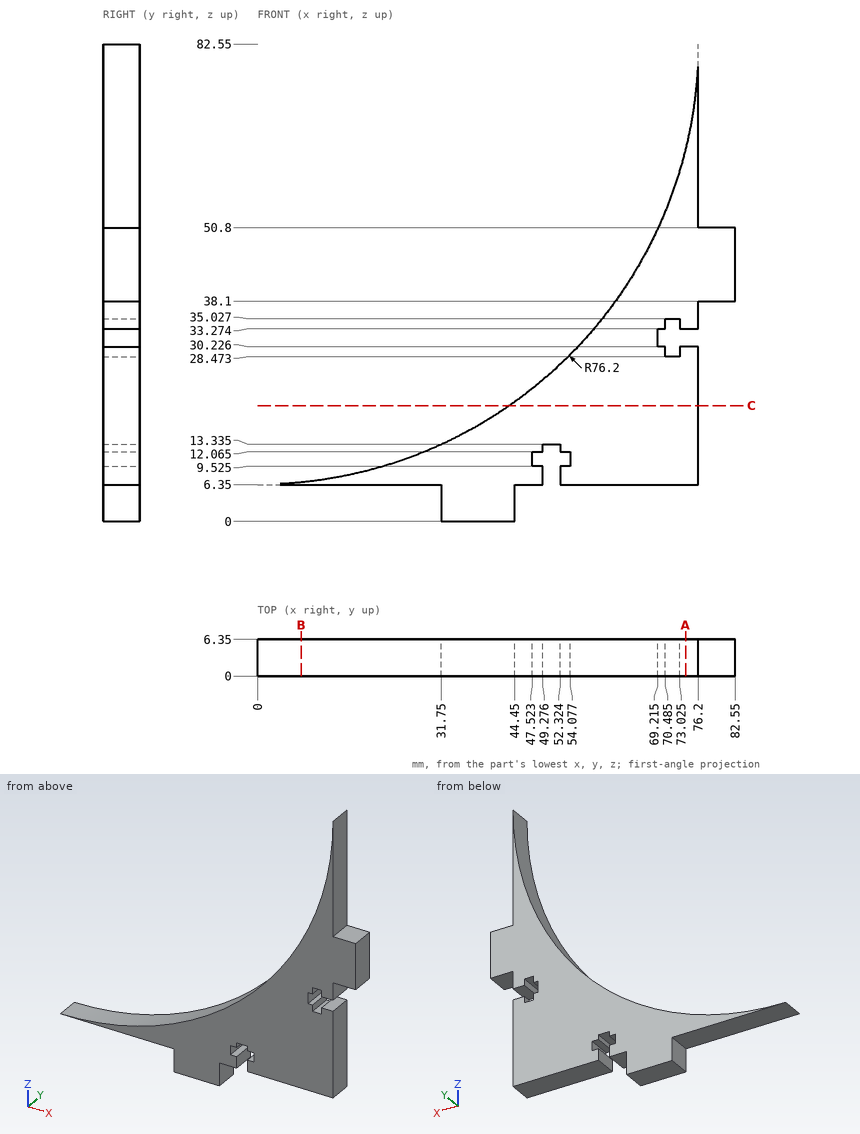
The drawing under review shows one solid part. Ordinate dimensions are in mm from its lowest x, y, z. Coordinates: 2 decimals unless noted, no trailing zeros. Order: outer loops, then holes, each group sorted by start corner. A loop starts at its lowest first (then second) coordinate and runs counter-clockwise, first axis right, second up. Notation, with made-up numbers: (87, 27.25) -> (146, 27.25) arc R19 ccw to (146, 64.25) -> close; hole circle Ø3 at (58.5, 37). An arc over 180 degrees is marked (long way). Answer in a Markdown table with one row per item. Add a question column.
Item 1: We need section A-A on x = 74. Write out the cut boundary in (y, z), plus the area to 3 significant figures.
Item 2: We need section C-C on z = 20. Write out the cut boundary in (x, y).
Item 3: Clearance check with flat-ended pins moving along their axes: pin 1 (1.6 mm diameter, centred on y = 4.5, z = 8, fed in from +X); pin 2 (0.5 mm diameter, centred on y = 4.5, z = 29.5, fed in from -X) (1 decimal); pin 3 (2.5 mm diameter, centred on x = 50, y = 2.5, fed in from -Z). State where each tip first meets the part, or that it passes through.
Item 4: We need section B-B on x = 7.5. Write out the cut boundary in (y, z).
Item 5: To check wall thickness, follow probe 1 along X at (y, z) = (1, 13) (1 decimal); probe 2 along X at (y, z) = (3.75, 70); probe 3 along Z at (x, y) = (58, 5.25). State the ranges of each line that lie inside material, in increasing order.
Final values:
| question | item | result |
|---|---|---|
| 1 | outline | (0, 6.35) -> (6.35, 6.35) -> (6.35, 30.23) -> (0, 30.23) -> close; (0, 33.27) -> (6.35, 33.27) -> (6.35, 64.37) -> (0, 64.37) -> close |
| 1 | area | 349 mm2 |
| 2 | outline | (43.52, 0) -> (76.2, 0) -> (76.2, 6.35) -> (43.52, 6.35) -> close |
| 3 | pin 1 | stops at x = 76.2 |
| 3 | pin 2 | stops at x = 54.5 |
| 3 | pin 3 | stops at z = 6.35 |
| 4 | outline | (0, 6.35) -> (6.35, 6.35) -> (6.35, 6.72) -> (0, 6.72) -> close |
| 5 | probe 1 | x = 31.1 to 49.3, 52.3 to 76.2 |
| 5 | probe 2 | x = 75.16 to 76.2 |
| 5 | probe 3 | z = 6.35 to 33.13 |
